Geometry: see drawing. Coordinates: mm, zero at the bounding-box minimum. A direction names the side the tool comes from. Coordinates: 2 decimals unless noted, no trailing zeros. Write each loop counter-clockwise with the first axis right and the second up, starting at its lowest first coordinate (ties: lowest second). Pieces come first, ordered by that corner, then holes.
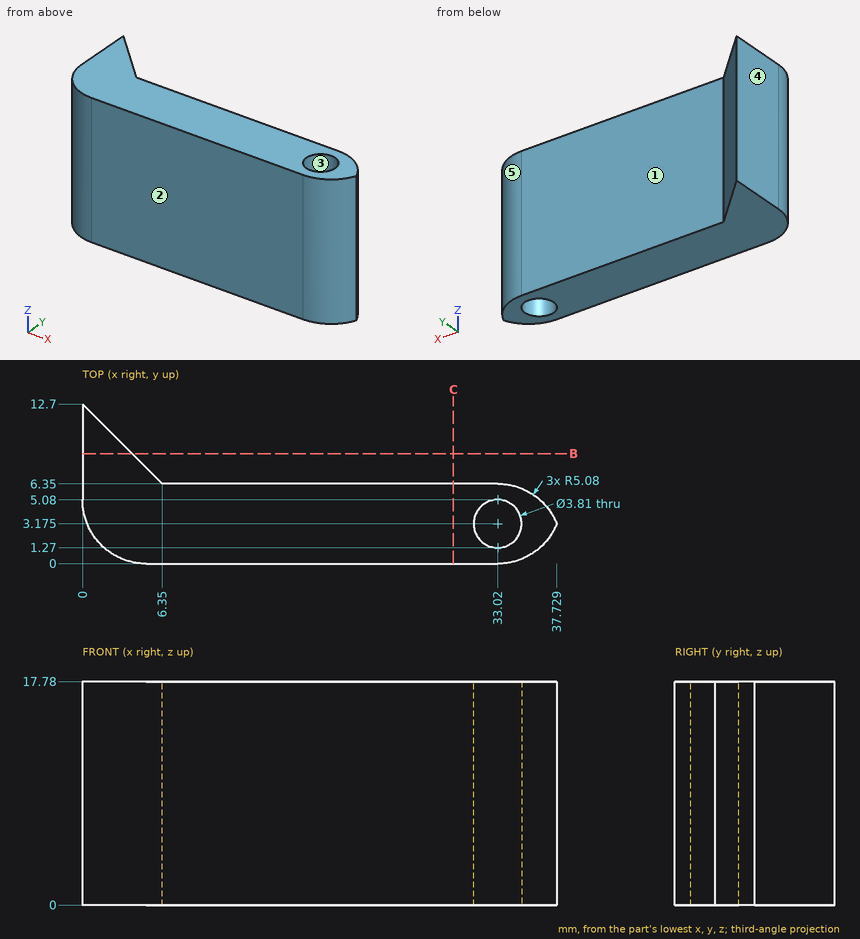
Item 1: Section B-B, the plane y = 8.75. Output: boundary loops of the cut face in (x, z).
Derived:
outline: (0, 0) - (3.95, 0) - (3.95, 17.78) - (0, 17.78) - close
Item 2: Set-up query: the marked faces 1 and 2. Return all of +Z, -Z, +X, -X, +Y, -Y with unobstructed straight access to the full face (end or side cutting, diameter ignored); none if empty.
Derived:
face 1: +Z, -Z, +X, +Y
face 2: +Z, -Z, +X, -X, -Y
Item 3: Material intervals for probe 1 along Y at (x, z) = (33.02, 8.75); probe 2 along X at (y, z) = (3.75, 12.5) (1 decimal); probe 3 along Y at (x, z) = (28, 4.5), sorted ascending.
Derived:
probe 1: y = 0 to 1.27, 5.08 to 6.35
probe 2: x = 0.2 to 31.2, 34.8 to 37.5
probe 3: y = 0 to 6.35
Item 4: Pin query (flat end, axial travel): pin 1 (4 mm diameter, centred on x = 22.5, z = 3, fed in from +Y). Return the tip coordinate at first contact, or that it passes through.
Derived:
pin 1: stops at y = 6.35
Item 5: Section C-C, the plane x = 29.5. Output: boundary loops of the cut face in (y, z).
Derived:
outline: (0, 0) - (6.35, 0) - (6.35, 17.78) - (0, 17.78) - close
Item 6: Pull-direction query (X, two-part tool) for the marked faces 3, 4 and 5; classes: released by +X, released by -X, zero draft, split by the parting line, or undercut.
Derived:
face 3: undercut
face 4: released by -X
face 5: released by +X
